Can you work these out from the model? Positions are in its coordinate system, mm. Give positions to 0.01 mm unless a question says otherwise; leave off trailing zeros. Order: outer loops, then holes, each group sorted by start corner. A loop starts at its lowest first (then second) coordinate and runs counter-clockwise, first axis right, second up. Notation, with made-up numbers: (1, 30.25) - (22, 30.25) arc R28 ccw to (22, 63.25) - close; hole circle Ø7 at (9, 7.25). An arc over 180 degrees is marked (long way). Answer as a JSON object with one key per item and string values.
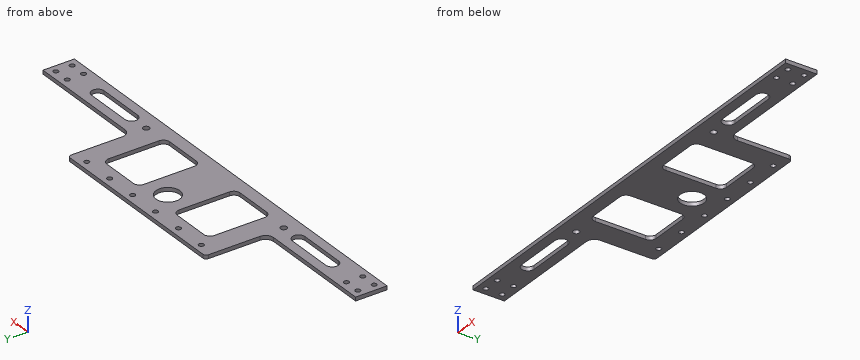
```python
from build123d import *

# Parameters (mm, degrees)
SKETCH1_R           = 9.5
SKETCH1_R_2         = 2
SKETCH1_R_3         = 2.5
BOSS_EXTRUDE1_DEPTH = 1.5


with BuildPart() as part:
    # Sketch1 → Boss-Extrude1 (new, symmetric)
    with BuildSketch(Plane.XY):
        with BuildLine():
            Line((177.5, 0), (177.5, 25))
            Line((177.5, 25), (84.5, 25))
            ThreePointArc((84.5, 25), (79.903805922, 26.903805922), (78, 31.5))
            Line((78, 31.5), (78, 72.5))
            ThreePointArc((78, 72.5), (77.267766953, 74.267766953), (75.5, 75))
            Line((75.5, 75), (-75.5, 75))
            ThreePointArc((-75.5, 75), (-77.267766953, 74.267766953), (-78, 72.5))
            Line((-78, 72.5), (-78, 31.5))
            ThreePointArc((-78, 31.5), (-79.903805922, 26.903805922), (-84.5, 25))
            Line((-84.5, 25), (-177.5, 25))
            Line((-177.5, 25), (-177.5, 0))
            Line((-177.5, 0), (177.5, 0))
        make_face()
        with Locations((0, 50)):
            Circle(SKETCH1_R, mode=Mode.SUBTRACT)
        with Locations((-65, 69)):
            Circle(SKETCH1_R_2, mode=Mode.SUBTRACT)
        with Locations((-39, 69)):
            Circle(SKETCH1_R_2, mode=Mode.SUBTRACT)
        with Locations((-13, 69)):
            Circle(SKETCH1_R_2, mode=Mode.SUBTRACT)
        with Locations((13, 69)):
            Circle(SKETCH1_R_2, mode=Mode.SUBTRACT)
        with Locations((39, 69)):
            Circle(SKETCH1_R_2, mode=Mode.SUBTRACT)
        with Locations((65, 69)):
            Circle(SKETCH1_R_2, mode=Mode.SUBTRACT)
        with Locations((-78, 12.5)):
            Circle(SKETCH1_R_3, mode=Mode.SUBTRACT)
        with Locations((-171.5, 19)):
            Circle(SKETCH1_R_2, mode=Mode.SUBTRACT)
        with Locations((-158.5, 19)):
            Circle(SKETCH1_R_2, mode=Mode.SUBTRACT)
        with Locations((-171.5, 6)):
            Circle(SKETCH1_R_2, mode=Mode.SUBTRACT)
        with Locations((-158.5, 6)):
            Circle(SKETCH1_R_2, mode=Mode.SUBTRACT)
        with Locations((171.5, 6)):
            Circle(SKETCH1_R_2, mode=Mode.SUBTRACT)
        with Locations((171.5, 19)):
            Circle(SKETCH1_R_2, mode=Mode.SUBTRACT)
        with Locations((158.5, 19)):
            Circle(SKETCH1_R_2, mode=Mode.SUBTRACT)
        with Locations((158.5, 6)):
            Circle(SKETCH1_R_2, mode=Mode.SUBTRACT)
        with Locations((78, 12.5)):
            Circle(SKETCH1_R_3, mode=Mode.SUBTRACT)
        with BuildLine():
            Line((-55, 60), (-25, 60))
            ThreePointArc((-25, 60), (-21.464466094, 58.535533906), (-20, 55))
            Line((-20, 55), (-20, 15))
            ThreePointArc((-20, 15), (-21.464466094, 11.464466094), (-25, 10))
            Line((-25, 10), (-55, 10))
            ThreePointArc((-55, 10), (-58.535533906, 11.464466094), (-60, 15))
            Line((-60, 15), (-60, 55))
            ThreePointArc((-60, 55), (-58.535533906, 58.535533906), (-55, 60))
        make_face(mode=Mode.SUBTRACT)
        with BuildLine():
            Line((-133, 17.5), (-95, 17.5))
            ThreePointArc((-95, 17.5), (-90, 12.5), (-95, 7.5))
            Line((-95, 7.5), (-133, 7.5))
            ThreePointArc((-133, 7.5), (-138, 12.5), (-133, 17.5))
        make_face(mode=Mode.SUBTRACT)
        with BuildLine():
            Line((133, 17.5), (95, 17.5))
            ThreePointArc((95, 17.5), (90, 12.5), (95, 7.5))
            Line((95, 7.5), (133, 7.5))
            ThreePointArc((133, 7.5), (138, 12.5), (133, 17.5))
        make_face(mode=Mode.SUBTRACT)
        with BuildLine():
            Line((55, 10), (25, 10))
            ThreePointArc((25, 10), (21.464466094, 11.464466094), (20, 15))
            Line((20, 15), (20, 55))
            ThreePointArc((20, 55), (21.464466094, 58.535533906), (25, 60))
            Line((25, 60), (55, 60))
            ThreePointArc((55, 60), (58.535533906, 58.535533906), (60, 55))
            Line((60, 55), (60, 15))
            ThreePointArc((60, 15), (58.535533906, 11.464466094), (55, 10))
        make_face(mode=Mode.SUBTRACT)
    extrude(amount=BOSS_EXTRUDE1_DEPTH, both=True)


solid = part.part
```
Q1. If we section it at A-A, the plane x = -110: Please give me the cut outline in (y, z).
Recorded:
{"outline": "(0, -1.5) - (7.5, -1.5) - (7.5, 1.5) - (0, 1.5) - close; (17.5, -1.5) - (25, -1.5) - (25, 1.5) - (17.5, 1.5) - close"}
Q2. I need wall thicknesses on L1, parallel to Y at x = -171.5, z = -0.2; L2, parallel to X at y = 34.5, z = -0.5; L3, parallel to X at y = 56, z = 1.15. Which ranges of each line are inside material? Lowest first, please.
Recorded:
{"L1": "y = 0 to 4, 8 to 17, 21 to 25", "L2": "x = -78 to -60, -20 to 20, 60 to 78", "L3": "x = -78 to -59.9, -20.1 to -7.37, 7.37 to 20.1, 59.9 to 78"}
Q3. I'm going to push flat-ended pins straight in: pin 1 Ø1 at (x, z) = (-87, 0.5) entering from -Y; pin 2 Ø6 at (x, y) = (25, 56) entering from +Z. Where does each tip first touch, or does it pass through?
Recorded:
{"pin 1": "stops at y = 0", "pin 2": "passes through"}
Q4. If we section it at B-B, the plane z = -0.35: Count the separate pieces of the cut face and the enclosed holes in it, then the cut area to 3 significant figures.
Recorded:
{"separate pieces": "1", "enclosed holes": "21", "area": "11,300 mm^2"}
